Read the model definition and answer for the solid it produces. Units are mm, in the model's axes. A direction names the side the tool comes from. Give positions to 0.01 mm unless a question says otherwise; leave off trailing zeros. Loops run counter-clockwise (first coordinate to the right, second up) from the corner with the lowest first, then second, coordinate; pieces in that order, holes last. Notation, with made-up numbers: (31.25, 45) -> (44.25, 45) arc R9 ccw to (44.25, 52) -> close; hole circle Ø3 at (-36, 7.5). An arc over 180 degrees is marked (long way). Return JSON: item names as keys, results as strings. Group by question number.
from build123d import *

# Parameters (mm, degrees)
F0_R     = 1
F1_DEPTH = 2
F2_R     = 1.95
F3_DEPTH = 1
F5_DEPTH = 30
F6_R     = 5
F7_DEPTH = 12.5


# Not quite as in the source:
# - ends of sketch curves that miss each other by under 0.0002 mm in the source are joined


with BuildPart() as f1:
    # F0 (on Top) → F1 (new body)
    with BuildSketch(Plane.XY):
        Polygon((0, -3), (0, 0), (0, 3), (-19, 1.5), (-19, 0), (-19, -1.5), align=None)
        with Locations((-14, 0)):
            Circle(F0_R, mode=Mode.SUBTRACT)
        Polygon((0, 3), (0, 0), (0, -3), (18.9999993891, -1.5), (18.9999993891, 0), (18.9999993891, 1.5), align=None)
        with Locations((14, 0)):
            Circle(F0_R, mode=Mode.SUBTRACT)
    extrude(amount=F1_DEPTH)

    # F2 (on face) → F3 (join)
    with BuildSketch(Plane.XY.offset(2)):
        Circle(F2_R)
    extrude(amount=F3_DEPTH)

    # F4 (on face) → F5 (join)
    with BuildSketch(Plane(origin=(0, 0, 0), x_dir=(1, 0, 0), z_dir=(0, 0, -1))):
        with BuildLine():
            Line((0, 3), (6.5447045484, 2.4833127822))
            ThreePointArc((6.5447045484, 2.4833127822), (9.2e-09, 7), (-6.5447045419, 2.4833127993))
            Line((-6.5447045419, 2.4833127993), (0, 3))
        make_face()
        with BuildLine():
            ThreePointArc((6.5447045484, -2.4833127822), (6.8852353569, -1.2623525976), (7, 0))
            ThreePointArc((7, 0), (6.8852353569, 1.2623525976), (6.5447045484, 2.4833127822))
            Line((6.5447045484, 2.4833127822), (0, 3))
            Line((0, 3), (-6.5447045419, 2.4833127993))
            ThreePointArc((-6.5447045419, 2.4833127993), (-7, 0), (-6.5447045419, -2.4833127993))
            Line((-6.5447045419, -2.4833127993), (0, -3))
            Line((0, -3), (6.5447045484, -2.4833127822))
        make_face()
        with BuildLine():
            ThreePointArc((-6.5447045419, -2.4833127993), (9.2e-09, -7), (6.5447045484, -2.4833127822))
            Line((6.5447045484, -2.4833127822), (0, -3))
            Line((0, -3), (-6.5447045419, -2.4833127993))
        make_face()
    extrude(amount=F5_DEPTH)

    # F6 (on Front) → F7 (cut, symmetric)
    with BuildSketch(Plane.XZ):
        with Locations((0, -20)):
            Circle(F6_R)
    extrude(amount=F7_DEPTH, both=True, mode=Mode.SUBTRACT)


solid = f1.part
1. Determine the mould class of faces 5 (the flat face through (0, 5, 0)), 6 (the cylindrical face through (-1.437, 1.318, 2.493)), 7 (the flat face through (12.7, 0, 0)), 8 (the cylindrical face through (4.619, -0.098, -21.915)) for opening direction Z: pulls with the +Z half, pulls with the -Z half, needs draft (parallel to the pull), parting line crosses it, or undercut.
2. Section C-C on y = 6 is taken. Determine the outline of the cut face in (x, z).
3. Straight lines are drawn through the part: line 1 (Z direction, x = 0, y = -4.5); line 2 (Y direction, x = 14, z = 1); line 3 (X direction, y = -0.25, z = -7.5). For each, find the intervals that lie inside material, in ascending order. Write a range as from..to.
4. Flat-ended cylindrical pins translate along their axes: pin 1 Ø2.5 at (x, y) = (-13, -1) entering from -Z; pin 2 Ø4 at (x, z) = (0.5, -26.5) entering from -Y; pin 3 Ø12 at (x, z) = (-9, -6) entering from -Y; pin 4 Ø5 at (x, y) = (-2.5, 4) entering from +Z. Find the tip coordinate at first contact, or state that the pin passes through.
5. Which of the six approach directions +Z, -Z, +X, -X, +Y, -Y give full straight-line access (tool end or side, diameter ignored) to faces 1 (the flat face through (9.63, 2.24, 0.99)), 2 (the flat face through (-9.63, -2.24, 0.99)), 3 (the flat face through (9.37, -2.26, 0.99)), 4 (the flat face through (-9.37, 2.26, 0.99))?
6. Section A-A on x = 2.5 is taken. Determine the outline of the cut face in (y, z), then the cut area to 3 significant figures.
7. Section D-D on z = -6.5 is taken. Determine the outline of the cut face in (x, y).
8. Section B-B on z = -20 is taken. Determine the outline of the cut face in (x, y), then the cut area to 3 significant figures.
Completed:
{
 "1": {"face 5": "pulls with the +Z half", "face 6": "needs draft", "face 7": "pulls with the -Z half", "face 8": "undercut"},
 "2": {"outline": "(-3.61, -30) -> (3.61, -30) -> (3.61, -23.46) arc R5 cw to (-3.61, -23.46) -> close; (-3.61, -16.54) arc R5 cw to (3.61, -16.54) -> (3.61, 0) -> (-3.61, 0) -> close"},
 "3": {"line 1": "z = -30..-25, -15..0", "line 2": "y = -1.89..-1, 1..1.89", "line 3": "x = -7..7"},
 "4": {"pin 1": "stops at z = 0", "pin 2": "stops at y = -7", "pin 3": "stops at y = -6.32", "pin 4": "stops at z = 2"},
 "5": {"face 1": "+Z, +X, +Y", "face 2": "+Z, -X, -Y", "face 3": "+Z, +X, -Y", "face 4": "+Z, -X, +Y"},
 "6": {"outline": "(-6.54, -30) -> (6.54, -30) -> (6.54, -24.33) -> (-6.54, -24.33) -> close; (-6.54, -15.67) -> (6.54, -15.67) -> (6.54, 0) -> (2.8, 0) -> (2.8, 2) -> (-2.8, 2) -> (-2.8, 0) -> (-6.54, 0) -> close", "area": "290 mm²"},
 "7": {"outline": "circle Ø14 at (0, 0)"},
 "8": {"outline": "(-5, -4.9) -> (-5, 4.9) arc R7 ccw to start; (5, -4.9) arc R7 ccw to (5, 4.9) -> close", "area": "27.0 mm²"}
}
